```python
from build123d import *

# Parameters (mm, degrees)
F2_R     = 2
F3_W     = 32
F3_H     = 45
F3_W_2   = 9
F3_H_2   = 20
F4_DEPTH = 3
F5_R     = 5
F6_R     = 2
F7_SIZE  = 0.5


with BuildPart() as f1:
    # F0 (on Front) → F1 (revolve)
    with BuildSketch(Plane.XZ):
        with BuildLine():
            ThreePointArc((0, 2.5), (2.5, 1.830127), (4.330127, 0))
            Line((4.330127, 0), (53, 0))
            Line((53, 0), (53, 5))
            Line((53, 5), (51, 5))
            Line((51, 5), (50.387579, 12))
            Line((50.387579, 12), (48.387579, 12))
            Line((48.387579, 12), (48.387579, 5))
            Line((48.387579, 5), (0, 5))
            Line((0, 5), (0, 2.5))
        make_face()
    revolve(axis=Axis((0, 0, 3.75), (0, 0, -1)))

    # F2
    f2_edges = [f1.edges().sort_by_distance(p)[0] for p in [
        (-53, 0, 0),
    ]]
    fillet(f2_edges, radius=F2_R)

    # F3 (on face) → F4 (cut)
    with BuildSketch(Plane.XY.offset(5)):
        Rectangle(F3_W, F3_H)
        Rectangle(F3_W_2, F3_H_2, mode=Mode.SUBTRACT)
    extrude(amount=-F4_DEPTH, mode=Mode.SUBTRACT)

    # F5
    f5_edges = [f1.edges().sort_by_distance(p)[0] for p in [
        (-16, 22.5, 3.5),
        (16, 22.5, 3.5),
        (16, -22.5, 3.5),
        (-16, -22.5, 3.5),
    ]]
    fillet(f5_edges, radius=F5_R)

    # F6
    f6_edges = [f1.edges().sort_by_distance(p)[0] for p in [
        (-4.5, 10, 3.5),
        (4.5, 10, 3.5),
        (4.5, -10, 3.5),
        (-4.5, -10, 3.5),
    ]]
    fillet(f6_edges, radius=F6_R)

    # F7
    f7_edges = [f1.edges().sort_by_distance(p)[0] for p in [
        (4.5, 0, 2),
        (0, 22.5, 2),
        (0, 22.5, 5),
    ]]
    chamfer(f7_edges, length=F7_SIZE)


solid = f1.part
```
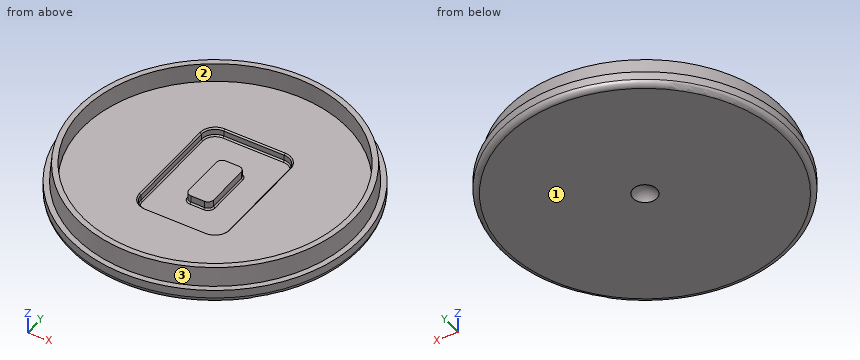
Here's how the part is built. I have some questions about the finished solid (model axes, mm). Face numbers are marked on the shaded views. Give positions to 0.01 mm unless a question says otherwise; leave off trailing zeros. Put each result on its own line as item: value. Start each with the question number.
Item 1: Thinking about a two-plate mould opening in Y: for the marked faces 1, 2 and 3, which applies, +Y half, -Y half, draft (parallel to the pull), parting line (faces both ways), or undercut?
Item 2: Will these pins go through, and if not, where does the flat tip stop? pin 1 (25 mm diameter, centred on x = 0, y = -3.5, fed in from +Z); pin 2 (1.6 mm diameter, centred on y = 5, z = 3, fed in from +X); pin 3 (1 mm diameter, centred on x = 1, z = 3.5, fed in from -Y).
Item 3: I need wall thicknesses on L1, parallel to X at y = 9, z = 2.5; L2, parallel to Y at x = -2.5, z = 3.5; L3, parallel to Y at x = 8.5, z = 9.75. Which ranges of each line are inside material? Lowest first, please. Write a range as from..to.
Values:
1. face 1: draft
1. face 2: undercut
1. face 3: parting line
2. pin 1: z = 5
2. pin 2: x = 52.83
2. pin 3: y = -53
3. L1: -52.23..-16, -4.23..4.23, 16..52.23
3. L2: -52.94..-22.5, -10..10, 22.5..52.94
3. L3: -49.87..-47.64, 47.64..49.87
